from build123d import *

# Parameters (mm, degrees)
ESQUISSE1_W                    = 6
ESQUISSE1_H                    = 42.7
ESQUISSE1_R                    = 0.95
BOSS_EXTRU_1_DEPTH             = 3
ESQUISSE2_W                    = 6
ESQUISSE2_H                    = 2.5
BOSS_EXTRU_2_DEPTH             = 6
BOSS_EXTRU_2_DIRECTION_2_REACH = 40.932
ESQUISSE3_W                    = 3
ESQUISSE3_H                    = 46.7
BOSS_EXTRU_4_DEPTH             = 44
ESQUISSE4_W                    = 9
ESQUISSE4_H                    = 2.5
BOSS_EXTRU_5_DEPTH             = 6
ENL_V_MAT_EXTRU_1_REACH        = 64.462
ESQUISSE5_R                    = 0.95
ENL_V_MAT_EXTRU_2_REACH        = 64.462
CONG_1_R                       = 5


with BuildPart() as part:
    # Esquisse1 → Boss.-Extru.1 (new body)
    with BuildSketch(Plane.XY):
        with Locations((0, 17.35)):
            Rectangle(ESQUISSE1_W, ESQUISSE1_H)
        Circle(ESQUISSE1_R, mode=Mode.SUBTRACT)
        with Locations((0, 34.7)):
            Circle(ESQUISSE1_R, mode=Mode.SUBTRACT)
    extrude(amount=BOSS_EXTRU_1_DEPTH)

    # Esquisse2 → Boss.-Extru.2 (add)
    with BuildSketch(Plane.XY.offset(3)):
        with Locations((0, 4.75)):
            Rectangle(ESQUISSE2_W, ESQUISSE2_H)
        with Locations((0, 39.45)):
            Rectangle(ESQUISSE2_W, ESQUISSE2_H)
        with Locations((0, 29.95)):
            Rectangle(ESQUISSE2_W, ESQUISSE2_H)
        with Locations((0, -4.75)):
            Rectangle(ESQUISSE2_W, ESQUISSE2_H)
    extrude(amount=BOSS_EXTRU_2_DEPTH)

    # Boss.-Extru.2 direction 2: up to this face of the body (flat: up to its plane)
    boss_extru_2_direction_2_end = Plane(part.part.faces().sort_by_distance((0, 17.35, 0))[0])
    # Esquisse2 → Boss.-Extru.2 direction 2 (add, up to the picked face)
    with BuildSketch(Plane.XY.offset(3), mode=Mode.PRIVATE) as boss_extru_2_direction_2_sk1:
        with Locations((0, 4.75)):
            Rectangle(ESQUISSE2_W, ESQUISSE2_H)
    boss_extru_2_direction_2_tool1 = split(extrude(boss_extru_2_direction_2_sk1.sketch, amount=-BOSS_EXTRU_2_DIRECTION_2_REACH, mode=Mode.PRIVATE), bisect_by=boss_extru_2_direction_2_end, keep=Keep.BOTH, mode=Mode.PRIVATE)
    # Esquisse2 → Boss.-Extru.2 direction 2 (add, up to the picked face)
    with BuildSketch(Plane.XY.offset(3), mode=Mode.PRIVATE) as boss_extru_2_direction_2_sk2:
        with Locations((0, 39.45)):
            Rectangle(ESQUISSE2_W, ESQUISSE2_H)
    boss_extru_2_direction_2_tool2 = split(extrude(boss_extru_2_direction_2_sk2.sketch, amount=-BOSS_EXTRU_2_DIRECTION_2_REACH, mode=Mode.PRIVATE), bisect_by=boss_extru_2_direction_2_end, keep=Keep.BOTH, mode=Mode.PRIVATE)
    # Esquisse2 → Boss.-Extru.2 direction 2 (add, up to the picked face)
    with BuildSketch(Plane.XY.offset(3), mode=Mode.PRIVATE) as boss_extru_2_direction_2_sk3:
        with Locations((0, 29.95)):
            Rectangle(ESQUISSE2_W, ESQUISSE2_H)
    boss_extru_2_direction_2_tool3 = split(extrude(boss_extru_2_direction_2_sk3.sketch, amount=-BOSS_EXTRU_2_DIRECTION_2_REACH, mode=Mode.PRIVATE), bisect_by=boss_extru_2_direction_2_end, keep=Keep.BOTH, mode=Mode.PRIVATE)
    # Esquisse2 → Boss.-Extru.2 direction 2 (add, up to the picked face)
    with BuildSketch(Plane.XY.offset(3), mode=Mode.PRIVATE) as boss_extru_2_direction_2_sk4:
        with Locations((0, -4.75)):
            Rectangle(ESQUISSE2_W, ESQUISSE2_H)
    boss_extru_2_direction_2_tool4 = split(extrude(boss_extru_2_direction_2_sk4.sketch, amount=-BOSS_EXTRU_2_DIRECTION_2_REACH, mode=Mode.PRIVATE), bisect_by=boss_extru_2_direction_2_end, keep=Keep.BOTH, mode=Mode.PRIVATE)
    add(boss_extru_2_direction_2_tool1.solids().sort_by(Axis((0, 4.75, 3), (0, 0, -1)))[0])
    add(boss_extru_2_direction_2_tool2.solids().sort_by(Axis((0, 39.45, 3), (0, 0, -1)))[0])
    add(boss_extru_2_direction_2_tool3.solids().sort_by(Axis((0, 29.95, 3), (0, 0, -1)))[0])
    add(boss_extru_2_direction_2_tool4.solids().sort_by(Axis((0, -4.75, 3), (0, 0, -1)))[0])

    # Esquisse3 → Boss.-Extru.4 (add)
    with BuildSketch(Plane.ZY.offset(3)):
        with Locations((1.5, 17.35)):
            Rectangle(ESQUISSE3_W, ESQUISSE3_H)
    extrude(amount=BOSS_EXTRU_4_DEPTH)

    # Esquisse4 → Boss.-Extru.5 (add)
    with BuildSketch(Plane.ZY.offset(47)):
        with Locations((4.5, 39.45)):
            Rectangle(ESQUISSE4_W, ESQUISSE4_H)
        with Locations((4.5, 29.95)):
            Rectangle(ESQUISSE4_W, ESQUISSE4_H)
        with Locations((4.5, 4.75)):
            Rectangle(ESQUISSE4_W, ESQUISSE4_H)
        with Locations((4.5, -4.75)):
            Rectangle(ESQUISSE4_W, ESQUISSE4_H)
    extrude(amount=-BOSS_EXTRU_5_DEPTH)

    # Esquisse5 → Enlèv. mat.-Extru.1 (cut, up to next)
    with BuildSketch(Plane.XY.offset(3), mode=Mode.PRIVATE) as enl_v_mat_extru_1_sk1:
        with Locations((-44, 34.7)):
            Circle(ESQUISSE5_R)
    enl_v_mat_extru_1_tool1 = extrude(enl_v_mat_extru_1_sk1.sketch, amount=-ENL_V_MAT_EXTRU_1_REACH, mode=Mode.PRIVATE) & part.part
    # Esquisse5 → Enlèv. mat.-Extru.1 (cut, up to next)
    with BuildSketch(Plane.XY.offset(3), mode=Mode.PRIVATE) as enl_v_mat_extru_1_sk2:
        with Locations((-44, 0)):
            Circle(ESQUISSE5_R)
    enl_v_mat_extru_1_tool2 = extrude(enl_v_mat_extru_1_sk2.sketch, amount=-ENL_V_MAT_EXTRU_1_REACH, mode=Mode.PRIVATE) & part.part
    add(enl_v_mat_extru_1_tool1.solids().sort_by_distance((-44, 34.7, 3))[0], mode=Mode.SUBTRACT)
    add(enl_v_mat_extru_1_tool2.solids().sort_by_distance((-44, 0, 3))[0], mode=Mode.SUBTRACT)

    # Esquisse6 → Enlèv. mat.-Extru.2 (cut, up to next)
    with BuildSketch(Plane.XY.offset(3), mode=Mode.PRIVATE) as enl_v_mat_extru_2_sk1:
        Polygon((-20.85, 20.35), (-23.15, 20.35), (-34, 31.2), (-10, 31.2), align=None)
    enl_v_mat_extru_2_tool1 = extrude(enl_v_mat_extru_2_sk1.sketch, amount=-ENL_V_MAT_EXTRU_2_REACH, mode=Mode.PRIVATE) & part.part
    # Esquisse6 → Enlèv. mat.-Extru.2 (cut, up to next)
    with BuildSketch(Plane.XY.offset(3), mode=Mode.PRIVATE) as enl_v_mat_extru_2_sk2:
        Polygon((-41, 28.7), (-41, 6), (-41, 3.5), (-27.15, 17.35), (-41, 31.2), align=None)
    enl_v_mat_extru_2_tool2 = extrude(enl_v_mat_extru_2_sk2.sketch, amount=-ENL_V_MAT_EXTRU_2_REACH, mode=Mode.PRIVATE) & part.part
    # Esquisse6 → Enlèv. mat.-Extru.2 (cut, up to next)
    with BuildSketch(Plane.XY.offset(3), mode=Mode.PRIVATE) as enl_v_mat_extru_2_sk3:
        Polygon((-3, 28.7), (-3, 6), (-3, 3.5), (-16.85, 17.35), (-3, 31.2), align=None)
    enl_v_mat_extru_2_tool3 = extrude(enl_v_mat_extru_2_sk3.sketch, amount=-ENL_V_MAT_EXTRU_2_REACH, mode=Mode.PRIVATE) & part.part
    # Esquisse6 → Enlèv. mat.-Extru.2 (cut, up to next)
    with BuildSketch(Plane.XY.offset(3), mode=Mode.PRIVATE) as enl_v_mat_extru_2_sk4:
        Polygon((-34, 3.5), (-23.15, 14.35), (-20.85, 14.35), (-10, 3.5), align=None)
    enl_v_mat_extru_2_tool4 = extrude(enl_v_mat_extru_2_sk4.sketch, amount=-ENL_V_MAT_EXTRU_2_REACH, mode=Mode.PRIVATE) & part.part
    # Esquisse6 → Enlèv. mat.-Extru.2 (cut, up to next)
    with BuildSketch(Plane.XY.offset(3), mode=Mode.PRIVATE) as enl_v_mat_extru_2_sk5:
        Polygon((-39.5, -2), (-41, -3.5), (-41, -6), (-3, -6), (-3, -3.5), (-4.5, -2), align=None)
    enl_v_mat_extru_2_tool5 = extrude(enl_v_mat_extru_2_sk5.sketch, amount=-ENL_V_MAT_EXTRU_2_REACH, mode=Mode.PRIVATE) & part.part
    # Esquisse6 → Enlèv. mat.-Extru.2 (cut, up to next)
    with BuildSketch(Plane.XY.offset(3), mode=Mode.PRIVATE) as enl_v_mat_extru_2_sk6:
        Polygon((-41, 40.7), (-41, 38.2), (-39.5, 36.7), (-4.5, 36.7), (-3, 38.2), (-3, 40.7), align=None)
    enl_v_mat_extru_2_tool6 = extrude(enl_v_mat_extru_2_sk6.sketch, amount=-ENL_V_MAT_EXTRU_2_REACH, mode=Mode.PRIVATE) & part.part
    add(enl_v_mat_extru_2_tool1.solids().sort_by_distance((-22, 27.267047, 3))[0], mode=Mode.SUBTRACT)
    add(enl_v_mat_extru_2_tool2.solids().sort_by_distance((-36.383333, 17.35, 3))[0], mode=Mode.SUBTRACT)
    add(enl_v_mat_extru_2_tool3.solids().sort_by_distance((-7.616667, 17.35, 3))[0], mode=Mode.SUBTRACT)
    add(enl_v_mat_extru_2_tool4.solids().sort_by_distance((-22, 7.432953, 3))[0], mode=Mode.SUBTRACT)
    add(enl_v_mat_extru_2_tool5.solids().sort_by_distance((-22, -4.022538, 3))[0], mode=Mode.SUBTRACT)
    add(enl_v_mat_extru_2_tool6.solids().sort_by_distance((-22, 38.722538, 3))[0], mode=Mode.SUBTRACT)

    # Congé1
    cong_1_edges = [part.edges().sort_by_distance(p)[0] for p in [
        (-44, 28.7, 3),
        (-44, 6, 3),
        (0, 6, 3),
        (0, 28.7, 3),
    ]]
    fillet(cong_1_edges, radius=CONG_1_R)


solid = part.part
Can you work these out from the model? Positions are in its coordinate system, mm. A direction names the side the tool comes from. Coordinates: 2 decimals unless noted, no trailing zeros. Write each loop counter-clockwise with the first axis right and the second up, starting at its lowest first coordinate (ties: lowest second). Pieces come first, ordered by that corner, then holes.
Q1. Please list where these lines run through material, in increasing order: L1, parallel to X at y = 34.7, z = 1.1; L2, parallel to X at y = 6, z = 1; L3, parallel to Y at x = -44, z = 2.1.
Results found:
L1: x = -47 to -44.95, -43.05 to -0.95, 0.95 to 3
L2: x = -47 to -41, -38.5 to -31.5, -12.5 to -5.5, -3 to 3
L3: y = -6 to -0.95, 0.95 to 33.75, 35.65 to 40.7
Q2. Which directions (+Z, -Z, +X, -X, +Y, -Y) give clear straight access to the entire face, cutting with the end or side of a thin tool? Please do faces 4 (the face through (-44, 3.5, 6)), 5 (the face through (-22, 36.7, 2)), 6 (the face through (-34, 24.2, 1.5)).
Results found:
face 4: +Z, +X, -X
face 5: +Z, -Z, +Y
face 6: +Z, -Z
Q3. If we mould it in two halves opening along X, with no side actions, what happens to faces 1 (the face through (-44, 31.2, 6)), 2 (the face through (-41, -5, 5)), 3 (the face through (-47, 23, 2))? For each: +X half, -X half, draft (parallel to the pull), parting line (faces both ways), or undercut.
Results found:
face 1: draft
face 2: undercut
face 3: -X half
Q4. Imagine slicing it at C-C, the plane x = 0. List the corners of the cut face in (y, z) for me, plus the area to 3 significant figures.
Results found:
outline: (-6, 0) - (-0.95, 0) - (-0.95, 3) - (-3.5, 3) - (-3.5, 9) - (-6, 9) - close; (0.95, 0) - (33.75, 0) - (33.75, 3) - (31.2, 3) - (31.2, 9) - (28.7, 9) - (28.7, 8) arc R5 cw to (23.7, 3) - (11, 3) arc R5 cw to (6, 8) - (6, 9) - (3.5, 9) - (3.5, 3) - (0.95, 3) - close; (35.65, 0) - (40.7, 0) - (40.7, 9) - (38.2, 9) - (38.2, 3) - (35.65, 3) - close
area: 199 mm2
Q5. For P1, Ø3, axis at x = -30, z = 3.5, coming from the +Y side; P2, Ø5, axis at x = -43, y = 20, coming from the +Z side; P3, Ø4, axis at x = -38, z = 3, coming from the -Y side, each with a flat end and sliding along its axis, tell me the tip position at first contact or that it passes through.
Results found:
P1: stops at y = 36.7
P2: stops at z = 3
P3: stops at y = -2.5
Q6. Imagine slicing it at D-D, the plane z = 5.5. Count the separate pieces of the cut face and the enclosed holes in it, plus the area to 3 significant figures.
Results found:
separate pieces: 8
enclosed holes: 0
area: 136 mm2
Q7. Imagine slicing it at A-A, the plane x = -7. List the corners of the cut face in (y, z) for me.
Results found:
outline: (-2, 0) - (7.5, 0) - (7.5, 3) - (-2, 3) - close; (27.2, 0) - (36.7, 0) - (36.7, 3) - (27.2, 3) - close
Q8. Imagine slicing it at B-B, the plane y = 0. List the corners of the cut face in (x, z) for me, plus the area to 3 significant figures.
Results found:
outline: (-47, 0) - (-44.95, 0) - (-44.95, 3) - (-47, 3) - close; (-43.05, 0) - (-0.95, 0) - (-0.95, 3) - (-43.05, 3) - close; (0.95, 0) - (3, 0) - (3, 3) - (0.95, 3) - close
area: 139 mm2
